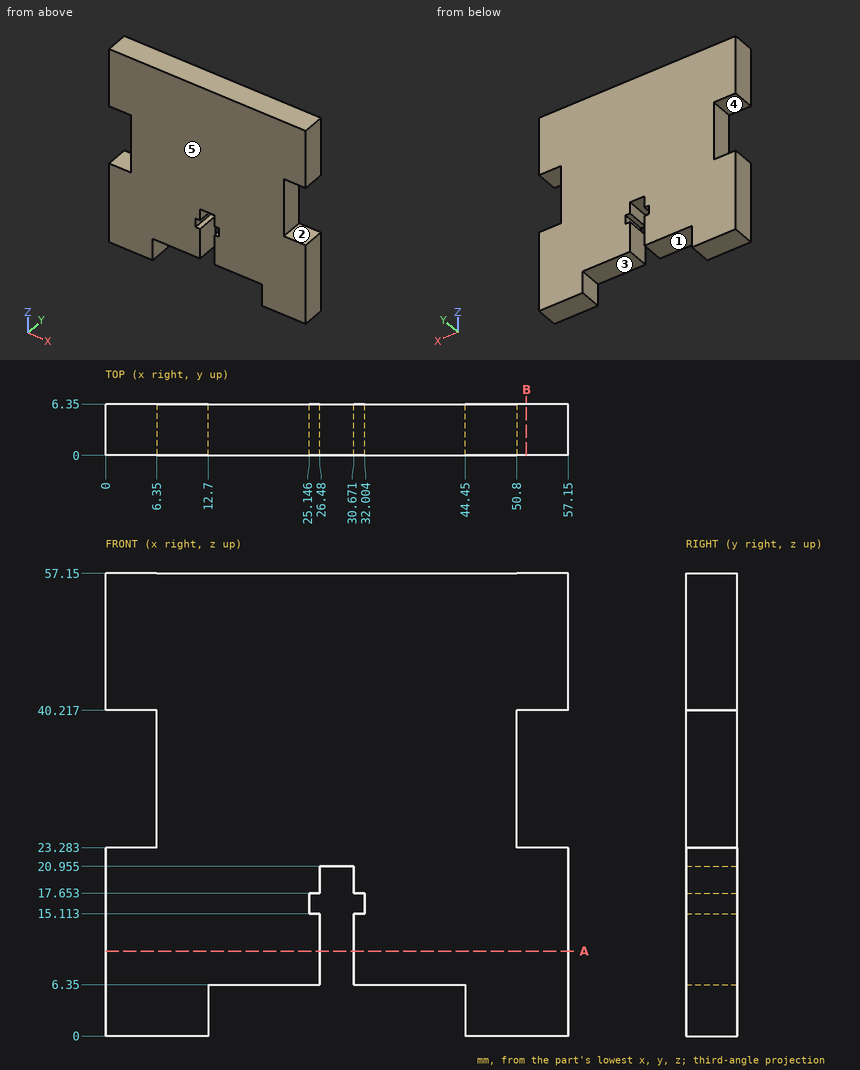
Here's the drawing with two shaded views (mm, measured from the low corner). I have some questions. A direction names the side the tool comes from. Coordinates: 2 decimals unless noted, no trailing zeros. Loops run counter-clockwise (first coordinate to the right, second up) from the corner with the lowest first, then second, coordinate; pieces in that order, holes last.
Item 1: Suppose I cut it at B-B (x = 52). Please give me the cut outline in (y, z).
Answers below:
outline: (0, 0) - (6.35, 0) - (6.35, 23.28) - (0, 23.28) - close; (0, 40.22) - (6.35, 40.22) - (6.35, 57.15) - (0, 57.15) - close
Item 2: Please list where these lines run through material, in increasing order: L1, parallel to X at y = 4, z = 20.5; L2, parallel to Z at x = 22.5, y = 5; L3, parallel to X at y = 4, z = 29.
Answers below:
L1: x = 0 to 26.48, 30.67 to 57.15
L2: z = 6.35 to 57.15
L3: x = 6.35 to 50.8
Item 3: Suppose I cut it at A-A (z = 10.5). Please give me the cut outline in (x, y), then the cut area to 3 significant figures.
Answers below:
outline: (0, 0) - (26.48, 0) - (26.48, 6.35) - (0, 6.35) - close; (30.67, 0) - (57.15, 0) - (57.15, 6.35) - (30.67, 6.35) - close
area: 336 mm2
Item 4: I'm going to push flat-ended pins straight in: pin 1 (1.5 mm diameter, centred on x = 31.5, y = 4, fed in from -Z); pin 2 (1.9 mm diameter, centred on y = 2.5, z = 31, fed in from +X); pin 3 (1.3 mm diameter, centred on x = 28, y = 2.5, fed in from -Z) (1 decimal). Where does each tip first touch, or does it pass through?
Answers below:
pin 1: stops at z = 6.35
pin 2: stops at x = 50.8
pin 3: stops at z = 21
Item 5: If we mould it in two halves opening along X, with no side actions, what happens to the marked faces 1, 2 and 3? For each: released by +X, released by -X, zero draft, split by the parting line, or undercut.
Answers below:
face 1: undercut
face 2: zero draft
face 3: undercut
Item 6: Which directions (+Z, -Z, +X, -X, +Y, -Y) give clear straight access to the entire face, cutting with the end or side of a thin tool? Please do the marked faces 4 and 5.
Answers below:
face 4: -X, +Y, -Y
face 5: +Z, -Z, +X, -X, -Y
